Read the model definition and answer for the solid it produces. Units are mm, in the model's axes. Coordinates: 2 decimals unless noted, no trailing zeros. Write each loop counter-clockwise with the first axis right and the second up, starting at its lowest first coordinate (ties: lowest second). Pieces come first, ordered by that corner, then holes. Notation, with made-up numbers: (6, 16.25) -> (14, 16.25) arc R26 ccw to (14, 50.25) -> close; hole circle Ø8 at (86.5, -17). An arc over 180 degrees is marked (long way). Use CSV: the item, a comma, the result in double quotes.
Autodesk Inventor part; units mm, degrees
ref_plane "Start Plane" through (0, 0, -9.7188) normal (0, 0, 1) x (1, 0, 0)
ref_plane "End Plane" through (0, 0, 142.7188) normal (0, 0, 1) x (1, 0, 0)
ref_plane "Work Plane4" through (2.3525, 9.2299, -7.9924) normal (-0.1588, -0.6229, -0.766) x (0.8923, -0.4227, 0.1588)
ref_plane "Start Plane" through (0, 0, -9.7188) normal (0, 0, 1) x (1, 0, 0)
ref_plane "End Plane" through (0, 0, 142.7188) normal (0, 0, 1) x (1, 0, 0)
sketch "Sketch" plane through (0, 0, 0) normal (0, 0, 1) x (1, 0, 0)
  circle A0 centre (0, 0) radius 9.525
  dimension "d0" = 19.05
extrude "Body" add sketch "Sketch" along normal up to surface (152.4376 mm away) from surface at -9.7188
sketch "Sketch2" plane through (0, 0, 0) normal (0, 0, 1) x (1, 0, 0)
  line L0 (0, 0) -> (10, 0)
ref_plane "Work Plane3" through (0, 0, 0) normal (0, -1, 0) x (1, 0, 0)
ref_plane "Work Plane4" through (2.3525, 9.2299, -7.9924) normal (-0.1588, -0.6229, -0.766) x (0.8923, -0.4227, 0.1588)
split "Split1" plane through (2.3525, 9.2299, -7.9924) removes the side toward (-0.1588, -0.6229, -0.766)
ref_plane "Work Plane5" through (2.3525, 9.2299, 140.9924) normal (-0.1588, -0.6229, 0.766) x (0.9857, -0.056, 0.1588)
split "Split2" plane through (2.3525, 9.2299, 140.9924) removes the side toward (-0.1588, -0.6229, 0.766)
sketch "Sketch3" plane through (0, 0, 0) normal (0, -1, 0) x (1, 0, 0)
  line L0 (-2, -9.7188) -> (12, -9.7188)
  line L1 (-2, 142.7188) -> (12, 142.7188)
  dimension "d7" = 152.4376
equation "\"d0\" = Diam"
equation "\"d1\" = G_L"
equation "\"Diam\" = 19.05"
equation "\"G_L\" = 148.98485"
equation "\"G_OFFSET_START\" = 9.71882"
equation "\"G_OFFSET_END\" = 9.71882"
equation "\"d4\" = -G_OFFSET_START"
equation "\"d5\" = G_OFFSET_END + B_L"
equation "\"B_L\" = 133"
properties part number "ANSI/AISC Rolled Steel - 3/4-5.866, RB" material "Steel, Mild"
1. Each of these flat-tipped pins is pushed along its axis until it touches: pin 1 Ø10 at (x, z) = (-7, 95.5) entering from +Y; pin 2 Ø3 at (x, y) = (7, 7) entering from +Z; pin 3 Ø8 at (x, z) = (5, 18.5) entering from +Y. Where does it stop, or does it pass through?
Solutions:
pin 1,"stops at y = 9.31"
pin 2,"stops at z = 140.4"
pin 3,"stops at y = 9.47"
2. A cutting plane is placed at C-C (x = -4.5). Give the vertices of the cut face in (y, z).
Solutions:
outline,"(-8.39, 7.76) -> (8.39, -5.89) -> (8.39, 138.89) -> (-8.39, 125.24) -> close"
3. A cutting plane is placed at B-B (y = 4.75). Give the vertices of the cut face in (x, z).
Solutions:
outline,"(-8.26, -2.15) -> (8.26, -5.57) -> (8.26, 138.57) -> (-8.26, 135.15) -> close"
4. Find the intervals of material crossed by line 1 along X through (y, z) = (-0.5, 96); line 2 along Y through (x, z) = (0.75, 63); line 3 along X through (y, z) = (3, 10), in increasing order.
Solutions:
line 1,"x = -9.51 to 9.51"
line 2,"y = -9.5 to 9.5"
line 3,"x = -9.04 to 9.04"
5. A cutting plane is placed at A-A (z = 47.5). Give the vertices of the cut face in (x, y) (3 decimals), and give its area (3 significant figures).
Solutions:
outline,"circle Ø19.05 at (0, 0)"
area,"285 mm^2"
